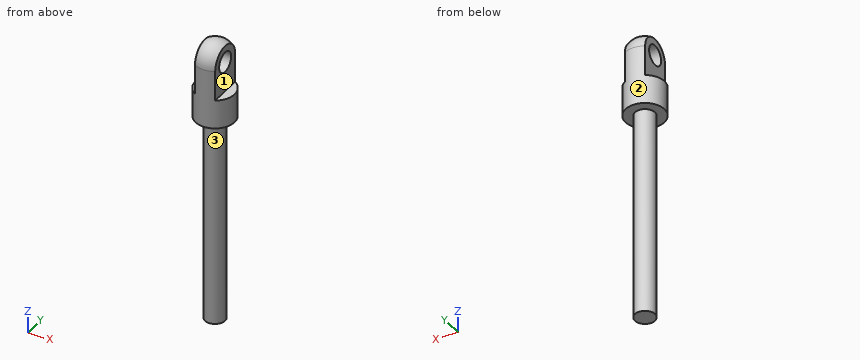
```python
from build123d import *

# Parameters (mm, degrees)
FILLET2_R               = 0.77724
SKETCH2_R               = 2.032
EXTRUDE2_DEPTH          = 2.032
SKETCH9_W               = 42.2148
SKETCH9_H               = 2.032
SKETCH12_R              = 2.032
CUT_EXTRUDE1_DEPTH      = 6.9690001
CUT_EXTRUDE1_DEPTH_BACK = 6.9690001
SKETCH13_OUTSIDE_W      = 37.724
SKETCH13_OUTSIDE_H      = 37.724
SKETCH13_OUTSIDE_W_2    = 4.064
SKETCH13_OUTSIDE_H_2    = 7.874
CUT_EXTRUDE2_DEPTH      = 4.937
CUT_EXTRUDE2_DEPTH_BACK = 6.096
LPATTERN1_COUNT         = 2
LPATTERN1_PITCH         = 29.972


with BuildPart() as part:
    # Sketch1 → Revolve1 (revolve)
    with BuildSketch(Plane(origin=(0, 0, 0), x_dir=(0, 0, -1), z_dir=(1, 0, 0))):
        Polygon((46.609, 0), (46.609, 5.969), (-13.0302, 5.969), (-13.0302, 2.0828), (16.9926, 2.0828), (29.1846, 2.0828), (29.1846, 0), align=None)
    revolve(axis=Axis((0, 0, 54.991), (0, 0, -1)))

    # Fillet2
    fillet2_edges = [part.edges().sort_by_distance(p)[0] for p in [
        (0, -5.969, 13.0302),
        (0, -5.969, -46.609),
    ]]
    fillet(fillet2_edges, radius=FILLET2_R)

    # Sketch2 → Extrude2 (add, symmetric)
    with BuildSketch(Plane(origin=(0, 0, 0), x_dir=(0, 0, -1), z_dir=(1, 0, 0))):
        with BuildLine():
            Line((46.609, 3.81), (54.991, 3.81))
            ThreePointArc((54.991, 3.81), (58.801, 0), (54.991, -3.81))
            Line((54.991, -3.81), (46.609, -3.81))
            Line((46.609, -3.81), (46.609, 3.81))
        make_face()
        with Locations((54.991, 0)):
            Circle(SKETCH2_R, mode=Mode.SUBTRACT)
    extrude(amount=EXTRUDE2_DEPTH, both=True)


with BuildPart() as body_2:
    # Sketch9 → Revolve5 (revolve)
    with BuildSketch(Plane(origin=(0, 0, 0), x_dir=(0, 0, -1), z_dir=(1, 0, 0))):
        with Locations((-21.9456, 1.016)):
            Rectangle(SKETCH9_W, SKETCH9_H)
    revolve(axis=Axis((0, 0, 43.053), (0, 0, 1)))

    # Sketch11 → Revolve6 (revolve)
    with BuildSketch(Plane(origin=(0, 0, 0), x_dir=(0, 0, -1), z_dir=(1, 0, 0))):
        with BuildLine():
            Line((-43.053, 0), (-43.053, 3.937))
            Line((-43.053, 3.937), (-54.991, 3.937))
            ThreePointArc((-54.991, 3.937), (-57.774879398, 2.783879398), (-58.928, 0))
            Line((-58.928, 0), (-43.053, 0))
        make_face()
    revolve(axis=Axis((0, 0, 58.928), (0, 0, 1)))

    # Sketch12 → Cut-Extrude1 (cut, two sides)
    with BuildSketch(Plane(origin=(0, 0, 0), x_dir=(0, 0, -1), z_dir=(1, 0, 0))) as cut_extrude1_sk:
        with Locations((-54.991, 0)):
            Circle(SKETCH12_R)
    extrude(amount=CUT_EXTRUDE1_DEPTH, mode=Mode.SUBTRACT)
    extrude(cut_extrude1_sk.sketch, amount=-CUT_EXTRUDE1_DEPTH_BACK, mode=Mode.SUBTRACT)

    # Sketch13 outside → Cut-Extrude2 (cut, two sides)
    with BuildSketch(Plane.XY.offset(54.991)) as cut_extrude2_sk:
        Rectangle(SKETCH13_OUTSIDE_W, SKETCH13_OUTSIDE_H)
        Rectangle(SKETCH13_OUTSIDE_W_2, SKETCH13_OUTSIDE_H_2, mode=Mode.SUBTRACT)
    extrude(amount=CUT_EXTRUDE2_DEPTH, mode=Mode.SUBTRACT)
    extrude(cut_extrude2_sk.sketch, amount=-CUT_EXTRUDE2_DEPTH_BACK, mode=Mode.SUBTRACT)


with BuildPart() as lpattern1_1:
    # LPattern1: pattern copy
    add(body_2.part.moved(Location(Vector(0, 0, -1) * (1 * LPATTERN1_PITCH))))


solid = lpattern1_1.part
```
Source: CAD feature listing. Evaluate the final solid. Frame: model axes, mm. Face numbers are marked on the shaded views. A direction names the side the tool comes from. Give positions to 0.01 mm unless a question says otherwise; leave off trailing zeros. Loops run counter-clockwise (first coordinate to the right, second up) from the corner with the lowest first, then second, coordinate; pieces in that order, holes last. Notation, with made-up numbers: M 70.5,-31.75 L 82.5,-31.75 A14 cw 82.5,-26.75 Z; hole C 4.5,39 d3. An arc over 180 degrees is marked long. Put each result on its own line as item: value.
Q1. Section C-C (z = -21.5). Return the cut outline in (x, y).
Response values:
outline: C 0,0 d4.06
Q2. Reachability of the marked faces 1, 2 and 3 from +Z, -Z, +X, -X, +Y, -Y: full face, straight path, thin tool, end or side. Return the list, or none.
Response values:
face 1: +Z, +X, +Y, -Y
face 2: +Z, -Z
face 3: -Z
Q3. Section B-B (x = 0.5). Return the cut outline in (y, z).
Response values:
outline: M -3.91,13.08 L -1.97,13.08 L -1.97,-29.13 L 1.97,-29.13 L 1.97,13.08 L 3.91,13.08 L 3.91,25.02 A3.91 ccw -3.91,25.02 Z; hole C 0,25.02 d4.06
Q4. Pin query (flat end, axial travel): P1, Ø3, axis at x = 3, z = 11.5, coming from the -Y side; P2, Ø2, axis at x = 1, z = -16.5, coming from the -Y side; P3, Ø4.5, axis at y = 0, z = 25.019, coming from the +X side; P4, Ø4, axis at x = 1.5, z = 23, coming from the -Y side. Return the tip coordinate at first contact, or that it passes through.
Response values:
P1: stops at y = -1.37
P2: stops at y = -2.03
P3: stops at x = 2.03
P4: stops at y = -3.94
Q5. Line query: probe 1 along Z at (x, y) = (3.75, 1); probe 2 along X at (y, z) = (2, 20.5); probe 3 along X at (y, z) = (-0.25, 18.5). Output: solid intervals per line, ascending. Write a range as [from, to].
Response values:
probe 1: z = [13.08, 18.92]
probe 2: x = [-2.03, 2.03]
probe 3: x = [-3.93, 3.93]
Q6. Section A-A (y = 0). Return the cut outline in (x, z), and give its area (3 significant figures).
Response values:
outline: M -3.94,13.08 L -2.03,13.08 L -2.03,-29.13 L 2.03,-29.13 L 2.03,13.08 L 3.94,13.08 L 3.94,18.92 L 2.03,18.92 L 2.03,22.99 L -2.03,22.99 L -2.03,18.92 L -3.94,18.92 Z; M -2.03,27.05 L 2.03,27.05 L 2.03,28.39 A3.94 ccw -2.03,28.39 Z
area: 241 mm²
